from build123d import *

# Parameters (mm, degrees)
EXTRUDE_1_DEPTH = 96


with BuildPart() as part:
    # Эскиз1 → Бобышка-Вытянуть1 (new body)
    with BuildSketch(Plane(origin=(0, 0, 0), x_dir=(1, 0, 0), z_dir=(0, 1, 0))):
        with BuildLine():
            Line((-46.843090279, -12.726935731), (-48.061840279, -13.004691807))
            Line((-48.061840279, -13.004691807), (-48.950659721, -9.104691807))
            Line((-48.950659721, -9.104691807), (-50.131159715, -9.373730613))
            ThreePointArc((-50.131159715, -9.373730613), (0, -51), (50.131159715, -9.373730613))
            Line((50.131159715, -9.373730613), (48.950659721, -9.104691807))
            Line((48.950659721, -9.104691807), (48.061840279, -13.004691807))
            Line((48.061840279, -13.004691807), (46.843090279, -12.726935731))
            Line((46.843090279, -12.726935731), (45.736038995, -17.584502752))
            ThreePointArc((45.736038995, -17.584502752), (0, -49), (-45.736038995, -17.584502752))
            Line((-45.736038995, -17.584502752), (-46.843090279, -12.726935731))
        make_face()
    extrude(amount=EXTRUDE_1_DEPTH)


solid = part.part
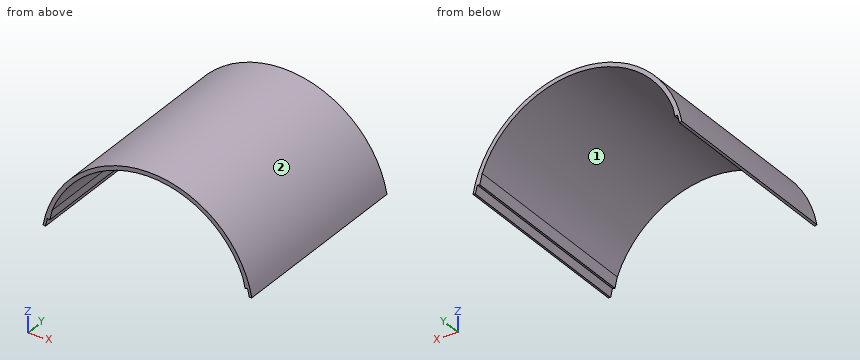
Part model, mm, in its own coordinate system. Face numbers are marked on the shaded views. Coordinates: 2 decimals unless noted, no trailing zeros. Order: outer loops, then holes, each group sorted by start corner. A loop starts at its lowest first (then second) coordinate and runs counter-clockwise, first axis right, second up. Notation, with made-up numbers: M 32,69.25 L 89,69.25 A16 ccw 89,87.25 Z; hole C -37,-6.75 d7. An arc over 180 degrees is marked long. Use a Markdown table: item, result.
(1) Cut at D-D on x = 26. Write the cut outline in (y, z).
A:
| item | result |
|---|---|
| outline | M 0,41.53 L 96,41.53 L 96,43.87 L 0,43.87 Z |
(2) Pull direction X, two halves, no side cores. Call the marked faces 1 and 2: released by +X, released by -X, zero draft, split by the parting line, or undercut.
A:
| item | result |
|---|---|
| face 1 | undercut |
| face 2 | split by the parting line |
(3) Flat gauge pins, fed straight in: pin 1 (3 mm diameter, centred on y = 12, z = 14, fed in from +X); pin 2 (1.5 mm diameter, centred on x = -10.5, y = 79.5, fed in from +Z); pin 3 (8 mm diameter, centred on y = 40, z = 30, fed in from -X). Where does each tip first touch, or does it go through?
A:
| item | result |
|---|---|
| pin 1 | stops at x = 49.44 |
| pin 2 | stops at z = 50.06 |
| pin 3 | stops at x = -43.87 |
(4) Cut at B-B on y = 23. Write the cut outline in (x, z).
A:
| item | result |
|---|---|
| outline | M -50.13,9.37 L -48.95,9.1 L -48.06,13 L -46.84,12.73 L -45.74,17.58 A49 cw 45.74,17.58 L 46.84,12.73 L 48.06,13 L 48.95,9.1 L 50.13,9.37 A51 ccw Z |
(5) Cut at A-A on z = 47. Write the cut outline in (x, y), then the cut area to 3 significant figures.
A:
| item | result |
|---|---|
| outline | M -19.8,0 L -13.86,0 L -13.86,96 L -19.8,96 Z; M 13.86,0 L 19.8,0 L 19.8,96 L 13.86,96 Z |
| area | 1,140 mm^2 |
(6) Probe L1, parallel to X at y = 28.5, z = 29.5; L2, parallel to X at y = 24, z = 36; L3, parallel to Z at x = 0, y = 71.5. List the from-to ranges inside material, lowest first.
A:
| item | result |
|---|---|
| L1 | x = -41.6 to -39.12, 39.12 to 41.6 |
| L2 | x = -36.12 to -33.24, 33.24 to 36.12 |
| L3 | z = 49 to 51 |
